For this review, take the finished solid that the model builds, in its own axes (mm). Face numbers are marked on the shaded views. Coordinates: 2 decimals unless noted, no trailing zeros. Order: outer loops, then holes, each group sorted by start corner. A loop starts at its lowest first (then second) coordinate and runs counter-clockwise, first axis right, second up. Notation, with made-up numbers: (27, -23.75) - (35, -23.75) arc R15 ccw to (35, -3.75) - close; hole circle Ø4 at (-24, 83.25). An arc over 180 degrees is marked (long way). One line per item, written item: value. Start each with the question number.
(1) Consider section A-A on x = -11. Write out the cut boundary in (y, z), then the cut area to 4 significant figures.
(2) To check wall thickness, follow line 1 along Y through (x, z) = (-38, 4.25); line 2 along X through (y, z) = (-3.5, 3.35); line 3 along Y through (x, z) = (-13.5, 0.8). State the ranges of each line that lie inside material, in increasing order.
(3) Consider section D-D on x = -36.5. Write out the cut boundary in (y, z).
(4) Consider section B-B on y = 8.5. Write out the cut boundary in (x, z).
(5) Clearance check with flat-ended pins moving along their axes: pin 1 (13 mm diameter, centred on x = -13.67, y = 6.75, fed in from -Z); pin 2 (5 mm diameter, centred on x = -14.5, y = -6.5, fed in from +Z); pin 3 (1.8 mm diameter, centred on x = -8.37, y = 23.25, fed in from +Z). State where each tip first meets the part, or that it passes through.
(6) Mouldability with a two-part tool opening along X and no side actions: class the marked faces 1 and 2 as released by +X, released by -X, zero draft, split by the parting line, or undercut.
(7) Consider section C-C on z = 2.9. Write out the cut boundary in (x, y), then the cut area to 3 significant figures.
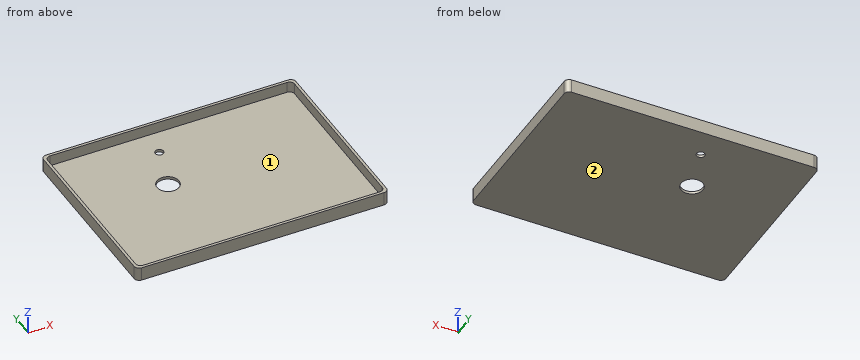
```python
from build123d import *

# Parameters (mm, degrees)
F0_W     = 92
F0_H     = 68
F0_W_2   = 90
F0_H_2   = 66
F2_DEPTH = 5
F3_DEPTH = 1
F1_R     = 4
F1_R_2   = 1.5
F4_DEPTH = 2.54
F5_R     = 1.8288


with BuildPart() as f2:
    # F0 (on Top) → F2 (new body)
    with BuildSketch(Plane.XY):
        Rectangle(F0_W, F0_H)
        Rectangle(F0_W_2, F0_H_2, mode=Mode.SUBTRACT)
    extrude(amount=F2_DEPTH)

    # F0 (on Top) → F3 (join)
    with BuildSketch(Plane.XY):
        Rectangle(F0_W_2, F0_H_2)
    extrude(amount=F3_DEPTH)

    # F1 (on Top) → F4 (cut)
    with BuildSketch(Plane.XY):
        with Locations((-13.673795, 6.754091)):
            Circle(F1_R)
        with Locations((-8.367444, 23.254091)):
            Circle(F1_R_2)
    extrude(amount=F4_DEPTH, mode=Mode.SUBTRACT)

    # F5
    f5_edges = [f2.edges().sort_by_distance(p)[0] for p in [
        (-45, 33, 3),
        (45, 33, 3),
        (-45, -33, 3),
        (45, -33, 3),
        (46, -34, 2.5),
        (-46, -34, 2.5),
        (-46, 34, 2.5),
        (46, 34, 2.5),
    ]]
    fillet(f5_edges, radius=F5_R)


solid = f2.part
```
Geometry check:
1. outline: (-34, 0) - (3.78, 0) - (3.78, 1) - (-33, 1) - (-33, 5) - (-34, 5) - close; (9.73, 0) - (34, 0) - (34, 5) - (33, 5) - (33, 1) - (9.73, 1) - close
1. area: 70.05 mm^2
2. line 1: y = -34 to -33, 33 to 34
2. line 2: x = -46 to -45, 45 to 46
2. line 3: y = -34 to 2.76, 10.75 to 34
3. outline: (-34, 0) - (34, 0) - (34, 5) - (33, 5) - (33, 1) - (-33, 1) - (-33, 5) - (-34, 5) - close
4. outline: (-46, 0) - (-17.27, 0) - (-17.27, 1) - (-45, 1) - (-45, 5) - (-46, 5) - close; (-10.07, 0) - (46, 0) - (46, 5) - (45, 5) - (45, 1) - (-10.07, 1) - close
5. pin 1: stops at z = 0
5. pin 2: stops at z = 1
5. pin 3: passes through
6. face 1: undercut
6. face 2: zero draft
7. outline: (-46, -32.17) arc R1.83 ccw to (-44.17, -34) - (44.17, -34) arc R1.83 ccw to (46, -32.17) - (46, 32.17) arc R1.83 ccw to (44.17, 34) - (-44.17, 34) arc R1.83 ccw to (-46, 32.17) - close; hole (-45, -31.17) arc R1.83 ccw to (-43.17, -33) - (43.17, -33) arc R1.83 ccw to (45, -31.17) - (45, 31.17) arc R1.83 ccw to (43.17, 33) - (-43.17, 33) arc R1.83 ccw to (-45, 31.17) - close
7. area: 316 mm^2
